from build123d import *
from OCP.BRepFilletAPI import BRepFilletAPI_MakeChamfer

# Parameters (mm, degrees)
SKETCH_1_R               = 10
EXTRUDE_1_DEPTH          = 2
SKETCH_2_R               = 10
SKETCH_2_R_2             = 8.5
EXTRUDE_2_DEPTH          = 3
SKETCH_4_R               = 13.5
SKETCH_4_R_2             = 8.5
EXTRUDE_3_DEPTH          = 1
SKETCH_5_R               = 12.25
SKETCH_5_R_2             = 8.5
EXTRUDE_4_DEPTH          = 8
SKETCH_6_R               = 0.9
CUT_EXTRUDE_1_DEPTH      = 8
SKETCH_7_R               = 3
SKETCH_7_R_2             = 1.15
CUT_EXTRUDE_2_DEPTH      = 24.674881204
CUT_EXTRUDE_3_DEPTH      = 24.674881204
CUT_EXTRUDE_3_DEPTH_BACK = 24.674881204
SKETCH_8_W               = 5
SKETCH_8_H               = 3
CUT_EXTRUDE_4_DEPTH      = 24.674881204
CUT_EXTRUDE_4_DEPTH_BACK = 24.674881204
SKETCH_9_W               = 3
SKETCH_9_H               = 5
EXTRUDE_5_DEPTH          = 3
CHAMFER_1_SIZE           = 0.2
CHAMFER_1_SIZE2          = 0.410060768


with BuildPart() as part:
    # 스케치1 → 보스-돌출1 (new body)
    with BuildSketch(Plane.XY):
        Circle(SKETCH_1_R)
    extrude(amount=EXTRUDE_1_DEPTH)

    # 스케치2 → 보스-돌출2 (add)
    with BuildSketch(Plane.XY.offset(2)):
        Circle(SKETCH_2_R)
        Circle(SKETCH_2_R_2, mode=Mode.SUBTRACT)
    extrude(amount=EXTRUDE_2_DEPTH)

    # 스케치4 → 보스-돌출3 (add)
    with BuildSketch(Plane.XY.offset(5)):
        Circle(SKETCH_4_R)
        Circle(SKETCH_4_R_2, mode=Mode.SUBTRACT)
    extrude(amount=EXTRUDE_3_DEPTH)

    # 스케치5 → 보스-돌출4 (add)
    with BuildSketch(Plane.XY.offset(6)):
        Circle(SKETCH_5_R)
        Circle(SKETCH_5_R_2, mode=Mode.SUBTRACT)
    extrude(amount=EXTRUDE_4_DEPTH)

    # 스케치6 → 컷-돌출1 (cut)
    with BuildSketch(Plane.XY.offset(14)):
        with Locations((10.375, 0)):
            Circle(SKETCH_6_R)
        with Locations((5.1875, -8.985013564)):
            Circle(SKETCH_6_R)
        with Locations((-5.1875, -8.985013564)):
            Circle(SKETCH_6_R)
        with Locations((-10.375, 0)):
            Circle(SKETCH_6_R)
        with Locations((-5.1875, 8.985013564)):
            Circle(SKETCH_6_R)
        with Locations((5.1875, 8.985013564)):
            Circle(SKETCH_6_R)
    extrude(amount=-CUT_EXTRUDE_1_DEPTH, mode=Mode.SUBTRACT)

    # 스케치7 → 컷-돌출2 (cut, through all)
    with BuildSketch(Plane(origin=(0, 0, 0), x_dir=(-1, 0, 0), z_dir=(0, 0, -1))):
        Circle(SKETCH_7_R)
        with Locations((-7, 0)):
            Circle(SKETCH_7_R_2)
        with Locations((7, 0)):
            Circle(SKETCH_7_R_2)
        with Locations((0, 7)):
            Circle(SKETCH_7_R_2)
        with Locations((0, -7)):
            Circle(SKETCH_7_R_2)
    extrude(amount=-CUT_EXTRUDE_2_DEPTH, mode=Mode.SUBTRACT)

    # 스케치8 → 컷-돌출3 (cut, two sides: drawn at the far end of the back side and taken through both)
    with BuildSketch(Plane(origin=(0, 0, 0), x_dir=(1, 0, 0), z_dir=(0, 1, 0)).offset(-CUT_EXTRUDE_3_DEPTH_BACK)):
        with Locations((0, -3.5)):
            Rectangle(SKETCH_8_W, SKETCH_8_H)
    extrude(amount=CUT_EXTRUDE_3_DEPTH + CUT_EXTRUDE_3_DEPTH_BACK, mode=Mode.SUBTRACT)

    # 스케치9 → 컷-돌출4 (cut, two sides: drawn at the far end of the back side and taken through both)
    with BuildSketch(Plane(origin=(0, 0, 0), x_dir=(0, 0, -1), z_dir=(1, 0, 0)).offset(-CUT_EXTRUDE_4_DEPTH_BACK)):
        with Locations((-3.5, 0)):
            Rectangle(SKETCH_9_W, SKETCH_9_H)
    extrude(amount=CUT_EXTRUDE_4_DEPTH + CUT_EXTRUDE_4_DEPTH_BACK, mode=Mode.SUBTRACT)

    # 스케치10 → 보스-돌출5 (add)
    with BuildSketch(Plane.XY.offset(14)):
        with BuildLine():
            Line((2.199961883, 8.210369523), (2.717599974, 10.142221176))
            ThreePointArc((2.717599974, 10.142221176), (0, 10.5), (-2.717599974, 10.142221176))
            Line((-2.717599974, 10.142221176), (-2.199961883, 8.210369523))
            ThreePointArc((-2.199961883, 8.210369523), (0, 8.5), (2.199961883, 8.210369523))
        make_face()
        with BuildLine():
            Line((6.01040764, 6.01040764), (7.424621202, 7.424621202))
            ThreePointArc((7.424621202, 7.424621202), (9.09326674, 5.25), (10.142221176, 2.717599974))
            Line((10.142221176, 2.717599974), (8.210369523, 2.199961883))
            ThreePointArc((8.210369523, 2.199961883), (7.361215932, 4.25), (6.01040764, 6.01040764))
        make_face()
        with BuildLine():
            Line((8.210369523, -2.199961883), (10.142221176, -2.717599974))
            ThreePointArc((10.142221176, -2.717599974), (9.09326674, -5.25), (7.424621202, -7.424621202))
            Line((7.424621202, -7.424621202), (6.01040764, -6.01040764))
            ThreePointArc((6.01040764, -6.01040764), (7.361215932, -4.25), (8.210369523, -2.199961883))
        make_face()
        with BuildLine():
            Line((2.199961883, -8.210369523), (2.717599974, -10.142221176))
            ThreePointArc((2.717599974, -10.142221176), (0, -10.5), (-2.717599974, -10.142221176))
            Line((-2.717599974, -10.142221176), (-2.199961883, -8.210369523))
            ThreePointArc((-2.199961883, -8.210369523), (0, -8.5), (2.199961883, -8.210369523))
        make_face()
        with BuildLine():
            Line((-6.01040764, -6.01040764), (-7.424621202, -7.424621202))
            ThreePointArc((-7.424621202, -7.424621202), (-9.09326674, -5.25), (-10.142221176, -2.717599974))
            Line((-10.142221176, -2.717599974), (-8.210369523, -2.199961883))
            ThreePointArc((-8.210369523, -2.199961883), (-7.361215932, -4.25), (-6.01040764, -6.01040764))
        make_face()
        with BuildLine():
            Line((-8.210369523, 2.199961883), (-10.142221176, 2.717599974))
            ThreePointArc((-10.142221176, 2.717599974), (-9.09326674, 5.25), (-7.424621202, 7.424621202))
            Line((-7.424621202, 7.424621202), (-6.01040764, 6.01040764))
            ThreePointArc((-6.01040764, 6.01040764), (-7.361215932, 4.25), (-8.210369523, 2.199961883))
        make_face()
    extrude(amount=EXTRUDE_5_DEPTH)

    # 모따기1: one chamfer whose edges measure the first distance from different faces: ONE call of the kernel's chamfer builder (chamfer() names one face for all edges)
    chamfer_1_edges_1 = [part.edges().sort_by_distance(p)[0] for p in [
        (-6.717514421, 6.717514421, 17),
    ]]
    chamfer_1_side_1 = [part.faces().sort_by_distance(p)[0] for p in [
        (-6.717514421, 6.717514421, 15.5),
    ]]
    chamfer_1_edges_2 = [part.edges().sort_by_distance(p)[0] for p in [
        (-9.09326674, 5.25, 17),
    ]]
    chamfer_1_side_2 = [part.faces().sort_by_distance(p)[0] for p in [
        (-9.09326674, 5.25, 15.5),
    ]]
    chamfer_1_edges_3 = [part.edges().sort_by_distance(p)[0] for p in [
        (-9.17629535, 2.458780928, 17),
    ]]
    chamfer_1_side_3 = [part.faces().sort_by_distance(p)[0] for p in [
        (-9.17629535, 2.458780928, 15.5),
    ]]
    chamfer_1_edges_4 = [part.edges().sort_by_distance(p)[0] for p in [
        (-9.17629535, -2.458780928, 17),
    ]]
    chamfer_1_side_4 = [part.faces().sort_by_distance(p)[0] for p in [
        (-9.17629535, -2.458780928, 15.5),
    ]]
    chamfer_1_edges_5 = [part.edges().sort_by_distance(p)[0] for p in [
        (-9.09326674, -5.25, 17),
    ]]
    chamfer_1_side_5 = [part.faces().sort_by_distance(p)[0] for p in [
        (-9.09326674, -5.25, 15.5),
    ]]
    chamfer_1_edges_6 = [part.edges().sort_by_distance(p)[0] for p in [
        (-6.717514421, -6.717514421, 17),
    ]]
    chamfer_1_side_6 = [part.faces().sort_by_distance(p)[0] for p in [
        (-6.717514421, -6.717514421, 15.5),
    ]]
    chamfer_1_edges_7 = [part.edges().sort_by_distance(p)[0] for p in [
        (0, 10.5, 17),
    ]]
    chamfer_1_side_7 = [part.faces().sort_by_distance(p)[0] for p in [
        (0, 10.5, 15.5),
    ]]
    chamfer_1_edges_8 = [part.edges().sort_by_distance(p)[0] for p in [
        (-2.458780928, 9.17629535, 17),
    ]]
    chamfer_1_side_8 = [part.faces().sort_by_distance(p)[0] for p in [
        (-2.458780928, 9.17629535, 15.5),
    ]]
    chamfer_1_edges_9 = [part.edges().sort_by_distance(p)[0] for p in [
        (2.458780928, 9.17629535, 17),
    ]]
    chamfer_1_side_9 = [part.faces().sort_by_distance(p)[0] for p in [
        (2.458780928, 9.17629535, 15.5),
    ]]
    chamfer_1_edges_10 = [part.edges().sort_by_distance(p)[0] for p in [
        (-2.458780928, -9.17629535, 17),
    ]]
    chamfer_1_side_10 = [part.faces().sort_by_distance(p)[0] for p in [
        (-2.458780928, -9.17629535, 15.5),
    ]]
    chamfer_1_edges_11 = [part.edges().sort_by_distance(p)[0] for p in [
        (0, -10.5, 17),
    ]]
    chamfer_1_side_11 = [part.faces().sort_by_distance(p)[0] for p in [
        (0, -10.5, 15.5),
    ]]
    chamfer_1_edges_12 = [part.edges().sort_by_distance(p)[0] for p in [
        (2.458780928, -9.17629535, 17),
    ]]
    chamfer_1_side_12 = [part.faces().sort_by_distance(p)[0] for p in [
        (2.458780928, -9.17629535, 15.5),
    ]]
    chamfer_1_edges_13 = [part.edges().sort_by_distance(p)[0] for p in [
        (9.09326674, 5.25, 17),
    ]]
    chamfer_1_side_13 = [part.faces().sort_by_distance(p)[0] for p in [
        (9.09326674, 5.25, 15.5),
    ]]
    chamfer_1_edges_14 = [part.edges().sort_by_distance(p)[0] for p in [
        (6.717514421, 6.717514421, 17),
    ]]
    chamfer_1_side_14 = [part.faces().sort_by_distance(p)[0] for p in [
        (6.717514421, 6.717514421, 15.5),
    ]]
    chamfer_1_edges_15 = [part.edges().sort_by_distance(p)[0] for p in [
        (9.17629535, 2.458780928, 17),
    ]]
    chamfer_1_side_15 = [part.faces().sort_by_distance(p)[0] for p in [
        (9.17629535, 2.458780928, 15.5),
    ]]
    chamfer_1_edges_16 = [part.edges().sort_by_distance(p)[0] for p in [
        (6.717514421, -6.717514421, 17),
    ]]
    chamfer_1_side_16 = [part.faces().sort_by_distance(p)[0] for p in [
        (6.717514421, -6.717514421, 15.5),
    ]]
    chamfer_1_edges_17 = [part.edges().sort_by_distance(p)[0] for p in [
        (9.09326674, -5.25, 17),
    ]]
    chamfer_1_side_17 = [part.faces().sort_by_distance(p)[0] for p in [
        (9.09326674, -5.25, 15.5),
    ]]
    chamfer_1_edges_18 = [part.edges().sort_by_distance(p)[0] for p in [
        (9.17629535, -2.458780928, 17),
    ]]
    chamfer_1_side_18 = [part.faces().sort_by_distance(p)[0] for p in [
        (9.17629535, -2.458780928, 15.5),
    ]]
    chamfer_1 = BRepFilletAPI_MakeChamfer(part.part.solid().wrapped)
    for e in chamfer_1_edges_1:
        chamfer_1.Add(CHAMFER_1_SIZE, CHAMFER_1_SIZE2, e.wrapped, chamfer_1_side_1[0].wrapped)  # the first distance lies on this face
    for e in chamfer_1_edges_2:
        chamfer_1.Add(CHAMFER_1_SIZE, CHAMFER_1_SIZE2, e.wrapped, chamfer_1_side_2[0].wrapped)  # the first distance lies on this face
    for e in chamfer_1_edges_3:
        chamfer_1.Add(CHAMFER_1_SIZE, CHAMFER_1_SIZE2, e.wrapped, chamfer_1_side_3[0].wrapped)  # the first distance lies on this face
    for e in chamfer_1_edges_4:
        chamfer_1.Add(CHAMFER_1_SIZE, CHAMFER_1_SIZE2, e.wrapped, chamfer_1_side_4[0].wrapped)  # the first distance lies on this face
    for e in chamfer_1_edges_5:
        chamfer_1.Add(CHAMFER_1_SIZE, CHAMFER_1_SIZE2, e.wrapped, chamfer_1_side_5[0].wrapped)  # the first distance lies on this face
    for e in chamfer_1_edges_6:
        chamfer_1.Add(CHAMFER_1_SIZE, CHAMFER_1_SIZE2, e.wrapped, chamfer_1_side_6[0].wrapped)  # the first distance lies on this face
    for e in chamfer_1_edges_7:
        chamfer_1.Add(CHAMFER_1_SIZE, CHAMFER_1_SIZE2, e.wrapped, chamfer_1_side_7[0].wrapped)  # the first distance lies on this face
    for e in chamfer_1_edges_8:
        chamfer_1.Add(CHAMFER_1_SIZE, CHAMFER_1_SIZE2, e.wrapped, chamfer_1_side_8[0].wrapped)  # the first distance lies on this face
    for e in chamfer_1_edges_9:
        chamfer_1.Add(CHAMFER_1_SIZE, CHAMFER_1_SIZE2, e.wrapped, chamfer_1_side_9[0].wrapped)  # the first distance lies on this face
    for e in chamfer_1_edges_10:
        chamfer_1.Add(CHAMFER_1_SIZE, CHAMFER_1_SIZE2, e.wrapped, chamfer_1_side_10[0].wrapped)  # the first distance lies on this face
    for e in chamfer_1_edges_11:
        chamfer_1.Add(CHAMFER_1_SIZE, CHAMFER_1_SIZE2, e.wrapped, chamfer_1_side_11[0].wrapped)  # the first distance lies on this face
    for e in chamfer_1_edges_12:
        chamfer_1.Add(CHAMFER_1_SIZE, CHAMFER_1_SIZE2, e.wrapped, chamfer_1_side_12[0].wrapped)  # the first distance lies on this face
    for e in chamfer_1_edges_13:
        chamfer_1.Add(CHAMFER_1_SIZE, CHAMFER_1_SIZE2, e.wrapped, chamfer_1_side_13[0].wrapped)  # the first distance lies on this face
    for e in chamfer_1_edges_14:
        chamfer_1.Add(CHAMFER_1_SIZE, CHAMFER_1_SIZE2, e.wrapped, chamfer_1_side_14[0].wrapped)  # the first distance lies on this face
    for e in chamfer_1_edges_15:
        chamfer_1.Add(CHAMFER_1_SIZE, CHAMFER_1_SIZE2, e.wrapped, chamfer_1_side_15[0].wrapped)  # the first distance lies on this face
    for e in chamfer_1_edges_16:
        chamfer_1.Add(CHAMFER_1_SIZE, CHAMFER_1_SIZE2, e.wrapped, chamfer_1_side_16[0].wrapped)  # the first distance lies on this face
    for e in chamfer_1_edges_17:
        chamfer_1.Add(CHAMFER_1_SIZE, CHAMFER_1_SIZE2, e.wrapped, chamfer_1_side_17[0].wrapped)  # the first distance lies on this face
    for e in chamfer_1_edges_18:
        chamfer_1.Add(CHAMFER_1_SIZE, CHAMFER_1_SIZE2, e.wrapped, chamfer_1_side_18[0].wrapped)  # the first distance lies on this face
    add(Compound.cast(chamfer_1.Shape()), mode=Mode.REPLACE)


solid = part.part
CAD build for the part. Positions are in the model's coordinates, mm. A direction names the side the tool comes from. Give positions to 0.01 mm unless a question says otherwise; leave off trailing zeros. Write each loop counter-clockwise with the first axis right and the second up, starting at its lowest first coordinate (ties: lowest second). Pieces come first, ordered by that corner, then holes. Notation, with made-up numbers: (-31.75, -34) - (-10.75, -34) arc R23 cw to (-10.75, -2) - close; hole circle Ø6 at (74, 30.5). An arc over 180 degrees is marked (long way). Put each result on its own line as item: value.
(1) Drop flat-ended pins along their axis: pin 1 Ø0.9 at (x, y) = (-10, -0.5) entering from +Z; pin 2 Ø15.5 at (x, y) = (0, 0) entering from +Z; pin 3 Ø1.4 at (x, y) = (-7, 0) entering from -Z; pin 4 Ø1 at (x, z) = (-2, 6) entering from +Y. Give the stop position or say it passes through.
Working result:
pin 1: z = 14
pin 2: z = 2
pin 3: through
pin 4: y = 13.42
(2) Saw through at B-B (x = 0). Count the separate pieces of the cut face and the enclosed holes in it, then the cut area to 3 significant figures.
Working result:
separate pieces: 6
enclosed holes: 0
area: 101 mm^2
(3) Tool access for faces 1 (the flat face through (9, 2.5, 4)), 2 (the cylindrical face through (-9.11, 5.22, 15.38)), 3 (the flat face through (-2.4, 2.4, 2)): list every direction of +Z, -Z, +X, -X, +Y, -Y with a clear straight run to the whole face (end or side of a thin tool).
Working result:
face 1: +X, -X
face 2: +Z, -X, +Y
face 3: none
(4) Pull direction Y, two halves, no side cores. Call faces 4 (the flat face through (-2.5, -9, 4)), 5 (the cylindrical face through (9.237, -3.83, 2.465)), 6 (the cylindrical face through (11.233, 0.27, 10.056)): released by +Y, released by -Y, zero draft, split by the parting line, or undercut.
Working result:
face 4: zero draft
face 5: split by the parting line
face 6: undercut
(5) Saw through at C-C (z = 2.75). List the corners of the cut face in (x, y).
Working result:
outline: (-9.68, -2.5) arc R10 ccw to (-2.5, -9.68) - (-2.5, -8.12) arc R8.5 cw to (-8.12, -2.5) - close; (-9.68, 2.5) - (-8.12, 2.5) arc R8.5 cw to (-2.5, 8.12) - (-2.5, 9.68) arc R10 ccw to start; (2.5, -9.68) arc R10 ccw to (9.68, -2.5) - (8.12, -2.5) arc R8.5 cw to (2.5, -8.12) - close; (2.5, 8.12) arc R8.5 cw to (8.12, 2.5) - (9.68, 2.5) arc R10 ccw to (2.5, 9.68) - close
(6) Saw through at D-D (y = 11.75). List the corners of the cut face in (x, z), then the cut area to 3 significant figures.
Working result:
outline: (-6.65, 5) - (6.65, 5) - (6.65, 6) - (3.46, 6) - (3.46, 14) - (-3.46, 14) - (-3.46, 6) - (-6.65, 6) - close
area: 68.7 mm^2
(7) Wall check: L1, parallel to X at y = -0.25, z = 7; L2, parallel to Z at x = 6.75, y = -4.5; L3, parallel to Z at x = -4.75, y = 11.25. Give the ranges that are in metal, low to high.
Working result:
L1: -12.25 to -11.24, -9.51 to -8.5, 8.5 to 9.51, 11.24 to 12.25
L2: 0 to 2
L3: 5 to 14
(8) Saw through at A-A (z = 14.75). List the corners of the cut face in (x, y).
Working result:
outline: (-10.14, -2.72) arc R10.5 ccw to (-7.42, -7.42) - (-6.01, -6.01) arc R8.5 cw to (-8.21, -2.2) - close; (-10.14, 2.72) - (-8.21, 2.2) arc R8.5 cw to (-6.01, 6.01) - (-7.42, 7.42) arc R10.5 ccw to start; (-2.72, -10.14) arc R10.5 ccw to (2.72, -10.14) - (2.2, -8.21) arc R8.5 cw to (-2.2, -8.21) - close; (-2.72, 10.14) - (-2.2, 8.21) arc R8.5 cw to (2.2, 8.21) - (2.72, 10.14) arc R10.5 ccw to start; (6.01, -6.01) - (7.42, -7.42) arc R10.5 ccw to (10.14, -2.72) - (8.21, -2.2) arc R8.5 cw to start; (6.01, 6.01) arc R8.5 cw to (8.21, 2.2) - (10.14, 2.72) arc R10.5 ccw to (7.42, 7.42) - close
